Print and shaded views of the part. All mm, measured from the part's lowest x, y and z. A direction names the side the tool comes from. Round coordinates to 2 decimals unless told otherwise and drop trailing zeros. Loops run counter-clockwise (first coordinate to the right, second up) from the corner with the lowest first, then second, coordinate; pieces in that order, holes last. Notation, with made-up numbers: (-39.75, 12) - (19.25, 12) arc R12 cw to (19.25, 27) - close; hole circle Ø7 at (-1, 24). An arc over 180 degrees is marked (long way). Answer as a JSON object with one key per item and string values.
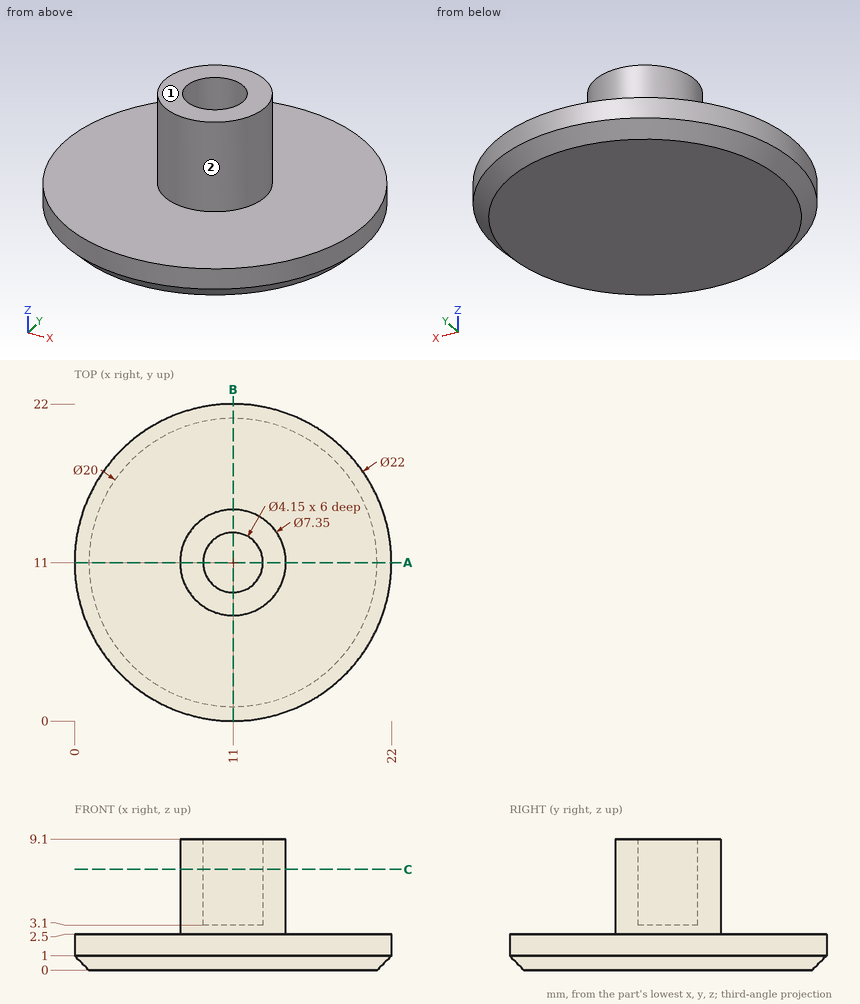
1) Slice it at A-A on y = 11. List the corners of the cut face in (x, z) (3 decimals).
Values follow:
{"outline": "(0, 1) - (1, 0) - (21, 0) - (22, 1) - (22, 2.5) - (14.675, 2.5) - (14.675, 9.1) - (13.075, 9.1) - (13.075, 3.1) - (8.925, 3.1) - (8.925, 9.1) - (7.325, 9.1) - (7.325, 2.5) - (0, 2.5) - close"}
2) Slice it at C-C on z = 7. List the corners of the cut face in (x, y) (3 decimals).
Values follow:
{"outline": "circle Ø7.35 at (11, 11); hole circle Ø4.15 at (11, 11)"}
3) Tool access for the marked faces 1 and 2: list every direction of +Z, -Z, +X, -X, +Y, -Y with a clear straight run to the whole face (end or side of a thin tool).
Values follow:
{"face 1": "+Z, +X, -X, +Y, -Y", "face 2": "+Z"}
4) Probe probe 1 along Y at (x, z) = (11, 6.25) (3 decimals); probe 2 along Z at (x, y) = (11.5, 17.75); probe 3 along Y at (x, z) = (12, 3.25). List the from-to ranges inside material, lowest first.
Values follow:
{"probe 1": "7.325 to 8.925, 13.075 to 14.675", "probe 2": "0 to 2.5", "probe 3": "7.46 to 9.18, 12.82 to 14.54"}
5) Drop flat-ended pins along their axis: P1, Ø2, axis at x = 16, y = 10.5, coming from the +Z side; P2, Ø3.5, axis at x = 10.5, y = 11.5, coming from the +Z side; P3, Ø3, axis at y = 9.5, z = 6.5, coming from the +X side (3 decimals); P4, Ø5, axis at x = 13.5, z = 6, coming from the -Y side (3 decimals). Give the stop position or say it passes through.
Values follow:
{"P1": "z = 2.5", "P2": "z = 9.1", "P3": "x = 14.675", "P4": "y = 7.325"}
